CAD build for the part. Positions are in the model's coordinates, mm. Round coordinates to 2 decimals unless told otherwise and drop trailing zeros. Use one line per item in the form item = value. Start each with the question number.
Item 1: Drill centre lines: L1, parallel to Y at x = 520, z = 0; L2, parallel to Y at x = 0, z = -4; L3, parallel to Y at x = 350, z = -0.75. Where is each one in solid material? Low to high.
Item 2: Pin check, flat tip, straight feed: pin 1 (5.5 mm diameter, centred on x = 521.5, y = -120, fed in from +Z). Stop position of the tip, or through.
Item 3: Pull direction Z, two halves, no side cores. Call faces 1 (the flat face through (-12, 2, 5)), 2 (the flat face through (-12, 2, -5)): +Z half, -Z half, draft (parallel to the pull), parting line (faces both ways), or undercut.
from build123d import *

# Parameters (mm, degrees)
SKETCH_1_W                          = 1700
SKETCH_1_H                          = 270
EXTRUDE_1_DEPTH                     = 5
HOLE_WIZARD_M6_1_AT_2_COUNT         = 2
HOLE_WIZARD_M6_1_AT_2_PITCH         = 250
HOLE_WIZARD_M6_1_AT_3_COUNT         = 2
HOLE_WIZARD_M6_1_AT_3_PITCH         = 125
HOLE_WIZARD_3_D                     = 6.6
HOLE_WIZARD_3_CBORE_D               = 11
HOLE_WIZARD_3_CBORE_DEPTH           = 6.8
PATTERN_LINEAR_1_COUNT              = 3
PATTERN_LINEAR_1_PITCH              = 25
PATTERN_LINEAR_1_COPY_1_D           = 6.6
PATTERN_LINEAR_1_COPY_1_CBORE_D     = 11
PATTERN_LINEAR_1_COPY_1_CBORE_DEPTH = 6.8
PATTERN_LINEAR_1_COPY_2_D           = 6.6
PATTERN_LINEAR_1_COPY_2_CBORE_D     = 11
PATTERN_LINEAR_1_COPY_2_CBORE_DEPTH = 6.8
HOLE_WIZARD_M5_1_D                  = 4.2
HOLE_WIZARD_3_2_D                   = 6.6
HOLE_WIZARD_3_2_CBORE_D             = 11
HOLE_WIZARD_3_2_CBORE_DEPTH         = 6.8
HOLE_WIZARD_3_3_D                   = 6.6
HOLE_WIZARD_3_3_CBORE_D             = 11
HOLE_WIZARD_3_3_CBORE_DEPTH         = 6.8
HOLE_WIZARD_M10_1_D                 = 8.5


with BuildPart() as part:
    # 草图1 → 凸台-拉伸1 (new body, symmetric)
    with BuildSketch(Plane.XY):
        Rectangle(SKETCH_1_W, SKETCH_1_H)
    extrude(amount=EXTRUDE_1_DEPTH, both=True)

    # 草图5 → M6 螺纹孔1 (revolve, cut)
    with BuildSketch(Plane(origin=(-850, 125, 0), x_dir=(0, 0, 1), z_dir=(0, 1, 0))):
        Polygon((0, 0), (0, 16.502151548), (2.5, 15), (2.5, 0), align=None)
    hole_wizard_m6_1 = revolve(axis=Axis((-856.35, 125, 0), (1, 0, 0)), mode=Mode.SUBTRACT)

    # M6 螺纹孔1 at 2: M6 螺纹孔1 ×2
    with Locations(*[(0, -i * HOLE_WIZARD_M6_1_AT_2_PITCH, 0) for i in range(1, HOLE_WIZARD_M6_1_AT_2_COUNT)]):
        add(hole_wizard_m6_1, mode=Mode.SUBTRACT)

    # M6 螺纹孔1 at 3: M6 螺纹孔1 ×2
    with Locations(*[(0, -i * HOLE_WIZARD_M6_1_AT_3_PITCH, 0) for i in range(1, HOLE_WIZARD_M6_1_AT_3_COUNT)]):
        add(hole_wizard_m6_1, mode=Mode.SUBTRACT)

    # 镜向1: M6 螺纹孔1 across plane
    add(hole_wizard_m6_1.mirror(Plane(origin=(0, 0, 0), x_dir=(0, 0, 1), z_dir=(1, 0, 0))), mode=Mode.SUBTRACT)

    # 镜向1 copy 1 sketch → 镜向1 copy 1 (revolve, cut)
    with BuildSketch(Plane(origin=(850, -125, 0), x_dir=(0, 0, 1), z_dir=(0, 1, 0))):
        Polygon((0, 0), (0, -16.502151548), (2.5, -15), (2.5, 0), align=None)
    revolve(axis=Axis((856.35, -125, 0), (1, 0, 0)), mode=Mode.SUBTRACT)

    # 镜向1 copy 2 sketch → 镜向1 copy 2 (revolve, cut)
    with BuildSketch(Plane(origin=(850, 0, 0), x_dir=(0, 0, 1), z_dir=(0, 1, 0))):
        Polygon((0, 0), (0, -16.502151548), (2.5, -15), (2.5, 0), align=None)
    revolve(axis=Axis((856.35, 0, 0), (1, 0, 0)), mode=Mode.SUBTRACT)

    # Hole Wizard 3 (through all)
    with Locations(Plane(origin=(-520, -70, 5), x_dir=(1, 0, 0), z_dir=(0, 0, 1))):
        with Locations((0, 0), (260, 0), (520, 0)):
            hole_wizard_3 = CounterBoreHole(HOLE_WIZARD_3_D / 2, HOLE_WIZARD_3_CBORE_D / 2, HOLE_WIZARD_3_CBORE_DEPTH)

    # 镜向4: Hole Wizard 3 across plane
    add(hole_wizard_3.mirror(Plane(origin=(0, 0, 0), x_dir=(0, 0, 1), z_dir=(1, 0, 0))), mode=Mode.SUBTRACT)

    # 阵列(线性)1: Hole Wizard 3 ×3
    with Locations(*[(0, -i * PATTERN_LINEAR_1_PITCH, 0) for i in range(1, PATTERN_LINEAR_1_COUNT)]):
        add(hole_wizard_3, mode=Mode.SUBTRACT)

    # 阵列(线性)1 copy 1 (through all)
    with Locations(Plane(origin=(520, -95, 5), x_dir=(-1, 0, 0), z_dir=(0, 0, 1))):
        with Locations((0, 0), (260, 0), (520, 0)):
            CounterBoreHole(PATTERN_LINEAR_1_COPY_1_D / 2, PATTERN_LINEAR_1_COPY_1_CBORE_D / 2, PATTERN_LINEAR_1_COPY_1_CBORE_DEPTH)

    # 阵列(线性)1 copy 2 (through all)
    with Locations(Plane(origin=(520, -120, 5), x_dir=(-1, 0, 0), z_dir=(0, 0, 1))):
        with Locations((0, 0), (260, 0), (520, 0)):
            CounterBoreHole(PATTERN_LINEAR_1_COPY_2_D / 2, PATTERN_LINEAR_1_COPY_2_CBORE_D / 2, PATTERN_LINEAR_1_COPY_2_CBORE_DEPTH)

    # M5 螺纹孔1 (through all)
    with Locations(Plane(origin=(-700, -10, 5), x_dir=(1, 0, 0), z_dir=(0, 0, 1))):
        with Locations((0, 0), (350, 0), (1400, 0), (1050, 0), (700, 0)):
            Hole(HOLE_WIZARD_M5_1_D / 2)

    # Hole Wizard 3 2 (through all)
    with Locations(Plane(origin=(835, 95, 5), x_dir=(1, 0, 0), z_dir=(0, 0, 1))):
        with Locations((0, 0)):
            CounterBoreHole(HOLE_WIZARD_3_2_D / 2, HOLE_WIZARD_3_2_CBORE_D / 2, HOLE_WIZARD_3_2_CBORE_DEPTH)

    # Hole Wizard 3 3 (through all)
    with Locations(Plane(origin=(-835, 95, 5), x_dir=(1, 0, 0), z_dir=(0, 0, 1))):
        with Locations((0, 0)):
            CounterBoreHole(HOLE_WIZARD_3_3_D / 2, HOLE_WIZARD_3_3_CBORE_D / 2, HOLE_WIZARD_3_3_CBORE_DEPTH)

    # M10 螺纹孔1 (through all)
    with Locations(Plane(origin=(-815, -90, 5), x_dir=(1, 0, 0), z_dir=(0, 0, 1))):
        with Locations((0, 0), (0, -30)):
            hole_wizard_m10_1 = Hole(HOLE_WIZARD_M10_1_D / 2)

    # 镜向5: M10 螺纹孔1 across plane
    add(hole_wizard_m10_1.mirror(Plane(origin=(0, 0, 0), x_dir=(0, 0, 1), z_dir=(1, 0, 0))), mode=Mode.SUBTRACT)


solid = part.part
Determined:
q1.L1 = -135 to -125.5, -114.5 to -100.5, -89.5 to -75.5, -64.5 to 135
q1.L2 = -135 to -123.3, -116.7 to -98.3, -91.7 to -73.3, -66.7 to -12.1, -7.9 to 135
q1.L3 = -135 to -12.1, -7.9 to 135
q2.pin_1 = -1.8
q3.face_1 = +Z half
q3.face_2 = -Z half
